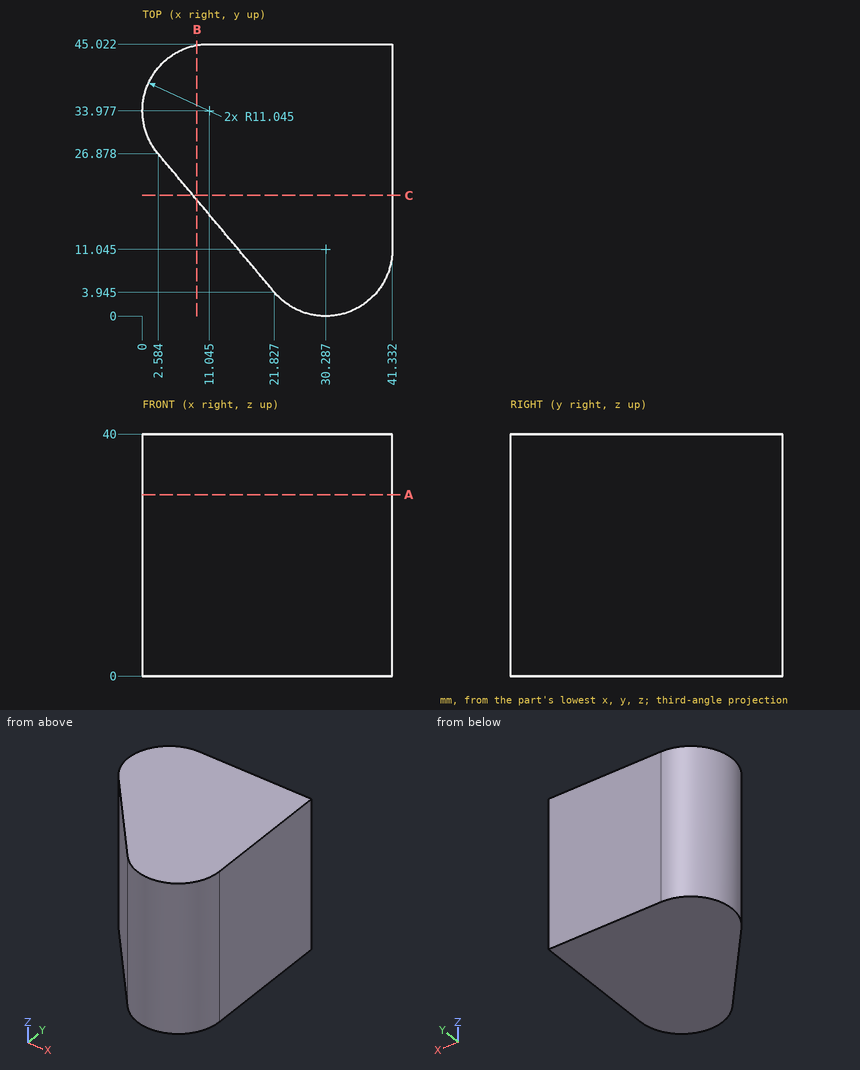
Here's the drawing with two shaded views (mm, measured from the low corner). I have some questions. Round coordinates to 2 decimals unless told otherwise and drop trailing zeros. Loops run counter-clockwise (first coordinate to the right, second up) from the corner with the lowest first, then second, coordinate; pieces in that order, holes last. Notation, with made-up numbers: M 81,89.5 L 118,89.5 A22 cw 118,105.5 Z; hole C 84,48.25 d2. An arc over 180 degrees is marked long. Answer as CSV lines item,"result".
1) Imagine slicing it at A-A on z = 30. List the corners of the cut face in (x, y) for me (1 decimal), and give its area (3 significant figures).
From the geometry:
outline,"M 2.6,26.9 L 21.8,3.9 A11 ccw 41.3,11 L 41.3,45 L 11,45 A11 ccw Z"
area,"1,430 mm^2"
2) For pin 1 Ø12 at (y, z) = (16.5, 34) entering from -X; pin 2 Ø1.5 at (x, z) = (10, 13.5) entering from -Y (1 decimal); pin 3 Ø10 at (y, z) = (21.5, 13.5) entering from -X, each with a flat end and sliding along its axis, tell me the tip position at first contact or that it passes through.
From the geometry:
pin 1,"x = 6.26"
pin 2,"y = 17.1"
pin 3,"x = 2.9"
3) If I drill on probe 1 along Y at (x, z) = (30.5, 5.5); probe 2 along X at (y, z) = (34, 23.5); probe 3 along X at (y, z) = (32, 24), over which ranges is the centre line in solid material (lowest first)?
From the geometry:
probe 1,"0 to 45.02"
probe 2,"0 to 41.33"
probe 3,"0.18 to 41.33"
4) Imagine slicing it at B-B on x = 9. List the corners of the cut face in (y, z) for me.
From the geometry:
outline,"M 19.23,0 L 44.83,0 L 44.83,40 L 19.23,40 Z"
5) Imagine slicing it at C-C on y = 20. List the corners of the cut face in (x, z) for me (1 decimal).
From the geometry:
outline,"M 8.4,0 L 41.3,0 L 41.3,40 L 8.4,40 Z"
